```python
from build123d import *

# Parameters (mm, degrees)
F1_DEPTH  = 50
F2_DEPTH  = 19
F4_DEPTH  = 10
F5_R      = 5
F6_R      = 8
F7_DEPTH  = 10
F9_R      = 19
F9_R_2    = 9
F10_DEPTH = 25
F11_DEPTH = 25
F12_W     = 10
F12_H     = 19
F13_DEPTH = 5
F14_DEPTH = 25
F15_R     = 15


with BuildPart() as f1:
    # F0 (on Front) → F1 (new body, symmetric)
    with BuildSketch(Plane.XZ):
        Polygon((0, 46), (0, 0), (68, 0), (68, 10), (10, 10), (10, 46), align=None)
    extrude(amount=F1_DEPTH, both=True)

    # F0 (on Front) → F2 (join, symmetric)
    with BuildSketch(Plane.XZ):
        Polygon((0, 46), (0, 0), (68, 0), (68, 10), (10, 10), (10, 46), align=None)
        Polygon((68, 10), (68, 0), (68, -29), (78, -29), (78, 10), align=None)
    extrude(amount=F2_DEPTH, both=True)

    # F3 (on face) → F4 (cut, through all)
    with BuildSketch(Plane.XY.offset(10)):
        with BuildLine():
            ThreePointArc((38.9489616917, -20.0184170119), (18.418397311, -29.1617077145), (10, -50))
            Line((10, -50), (68, -50))
            Line((68, -50), (68, -19))
            Line((68, -19), (38.9489616917, -20.0184170119))
        make_face()
        with BuildLine():
            Line((68, 50), (10, 50))
            ThreePointArc((10, 50), (18.418397311, 29.1617077145), (38.9489616917, 20.0184170119))
            Line((38.9489616917, 20.0184170119), (68, 19))
            Line((68, 19), (68, 50))
        make_face()
    extrude(amount=-F4_DEPTH, mode=Mode.SUBTRACT)

    # F5
    f5_edges = [f1.edges().sort_by_distance(p)[0] for p in [
        (68, 0, 0),
    ]]
    fillet(f5_edges, radius=F5_R)

    # F6 (on face) → F7 (cut)
    with BuildSketch(Plane.YZ.offset(10)):
        with Locations((-30, 28)):
            Circle(F6_R)
        with Locations((30, 28)):
            Circle(F6_R)
    extrude(amount=-F7_DEPTH, mode=Mode.SUBTRACT)

    # F9 (on offset) → F10 (join)
    with BuildSketch(Plane.YZ.offset(90)):
        with Locations((0, -29)):
            Circle(F9_R)
        with Locations((0, -29)):
            Circle(F9_R_2, mode=Mode.SUBTRACT)
    extrude(amount=-F10_DEPTH)

    # F11 (cut): a face of the model
    f11_faces = [f1.faces().sort_by_distance(p)[0] for p in [
        (78, 0, -25.1802813658),
    ]]
    extrude(f11_faces, amount=-F11_DEPTH, mode=Mode.SUBTRACT)

    # F12 (on Front) → F13 (join, symmetric)
    with BuildSketch(Plane.XZ):
        with BuildLine():
            ThreePointArc((39.7321374946, 20), (19.9837198365, 27.4168204187), (10, 46))
            Line((10, 46), (10, 10))
            Line((10, 10), (38.9489616917, 10))
            Line((38.9489616917, 10), (68, 10))
            Line((68, 10), (73, 10))
            ThreePointArc((73, 10), (76.5355339059, 8.5355339059), (78, 5))
            Line((78, 5), (78, -10))
            Line((78, -10), (88, -10))
            ThreePointArc((88, -10), (79.2132034356, 11.2132034356), (58, 20))
            Line((58, 20), (39.7321374946, 20))
        make_face()
        with BuildLine():
            Line((73, 10), (68, 10))
            Line((68, 10), (68, -5))
            Line((68, -5), (68, -10))
            Line((68, -10), (78, -10))
            Line((78, -10), (78, 5))
            ThreePointArc((78, 5), (76.5355339059, 8.5355339059), (73, 10))
        make_face()
        with Locations((83, -19.5)):
            Rectangle(F12_W, F12_H)
        with Locations((73, -19.5)):
            Rectangle(F12_W, F12_H)
    extrude(amount=F13_DEPTH, both=True)

    # F14 (cut): a face of the model
    f14_faces = [f1.faces().sort_by_distance(p)[0] for p in [
        (88, 0, -24.7319215604),
    ]]
    extrude(f14_faces, amount=-F14_DEPTH, mode=Mode.SUBTRACT)

    # F15
    f15_edges = [f1.edges().sort_by_distance(p)[0] for p in [
        (78, -12, 10),
        (78, 12, 10),
    ]]
    fillet(f15_edges, radius=F15_R)


solid = f1.part
```
Geometry check sheet. Reference: the model listing, model coordinates, mm. A direction names the side the tool comes from. Round coordinates to 2 decimals unless told otherwise and drop trailing zeros. Order: outer loops, then holes, each group sorted by start corner. A loop starts at its lowest first (then second) coordinate and runs counter-clockwise, first axis right, second up. Notation, with made-up numbers: (0, 1) -> (48, 1) arc R21 cw to (48, 28) -> close; hole circle Ø3 at (-6.5, 33.5). An arc over 180 degrees is marked (long way). Return JSON: item names as keys, results as strings. Group by question number.
Q1. Section check B-B, the plane y = 30. Record the boundary of the cut face in (x, z), plus the area to 3 significant figures.
Q2. Section check C-C, the plane z = 22. Record the boundary of the cut face in (x, y).
Q3. Section check D-D, the plane x = 34.5. Record the boundary of the cut face in (y, z).
Q4. Release check for a two-part mould opening along Y. For faces 4 (the cylindrical face through (5.1, 24.1, 33.4)), 5 (the cylindrical face through (5, -38, 28)), 6 (the flat face through (10, 22, 32)), 7 (the flat face through (5, 50, 23)) record: released by +Y, released by -Y, zero draft, split by the parting line, or undercut.
Q5. Gauge pin test, flat ends, axial feed: pin 1 (11.5 mm diameter, centred on y = 6, z = -31.5, fed in from -X); pin 2 (3 mm diameter, centred on x = 32.5, z = 15.5, fed in from +Y); pin 3 (8 mm diameter, centred on x = 46, y = -2, fed in from +Z). Record the tip position at first contact, or that the pin passes through.
Q6. Section check A-A, the plane z = 34. Record the boundary of the cut face in (x, y).
Q7. Material ranges on probe 1 along Z at (x, y) = (6, 30); probe 2 along Y at (x, z) = (71, -14); probe 3 along X at (y, z) = (-12, -28), recorded low to high. Write a range as from..to.
Q8. Tool access check on faces 1 (the cylindrical face through (73.49, 11.99, 5.72)), 2 (the flat face through (24, -1, 0)), 3 (the flat face through (31, -13, 10)). Record the directions out of +Z, -Z, +X, -X, +Y, -Y that give a thin tool (end or side, any length) a straight path to the whole face; none if there is none.
Numbers:
{
 "1": {"outline": "(0, 0) -> (17.64, 0) -> (17.64, 10) -> (10, 10) -> (10, 20) -> (0, 20) -> close; (0, 36) -> (10, 36) -> (10, 46) -> (0, 46) -> close", "area": "376 mm^2"},
 "2": {"outline": "(0, -50) -> (10, -50) -> (10, -35.29) -> (0, -35.29) -> close; (0, -24.71) -> (10, -24.71) -> (10, -5) -> (28.96, -5) -> (28.96, 5) -> (10, 5) -> (10, 24.71) -> (0, 24.71) -> close; (0, 35.29) -> (10, 35.29) -> (10, 50) -> (0, 50) -> close"},
 "3": {"outline": "(-20.51, 0) -> (20.51, 0) -> (20.51, 10) -> (5, 10) -> (5, 20.46) -> (-5, 20.46) -> (-5, 10) -> (-20.51, 10) -> close"},
 "4": {"face 4": "undercut", "face 5": "undercut", "face 6": "zero draft", "face 7": "released by +Y"},
 "5": {"pin 1": "x = 65", "pin 2": "y = 5", "pin 3": "z = 20"},
 "6": {"outline": "(0, -50) -> (10, -50) -> (10, -35.29) -> (0, -35.29) -> close; (0, -24.71) -> (10, -24.71) -> (10, -5) -> (14.35, -5) -> (14.35, 5) -> (10, 5) -> (10, 24.71) -> (0, 24.71) -> close; (0, 35.29) -> (10, 35.29) -> (10, 50) -> (0, 50) -> close"},
 "7": {"probe 1": "0..20, 36..46", "probe 2": "-19..19", "probe 3": "65..90"},
 "8": {"face 1": "+Z, +X, +Y", "face 2": "-Z, -X, +Y, -Y", "face 3": "+Z, +X, -Y"}
}
